Autodesk Inventor part; units mm, degrees
ref_plane "РабПлоскость1" through (0, 0, 75.2) normal (0, 0, 1) x (1, 0, 0)
ref_plane "YZ Plane" through (0, 0, 0) normal (1, 0, 0) x (0, 1, 0)
ref_plane "XZ Plane" through (0, 0, 0) normal (0, 1, 0) x (-1, 0, 0)
ref_plane "РабПлоскость1" through (0, 0, 75.2) normal (0, 0, 1) x (1, 0, 0)
sketch "Эскиз1" plane through (0, 0, 75.2) normal (0, 0, 1) x (1, 0, 0)
  circle A0 centre (26.4645, -26.4645) radius 1.95 construction
  circle A1 centre (-26.4645, 26.4645) radius 1.95 construction
  circle A2 centre (26.4645, 26.4645) radius 1.95 construction
  circle A3 centre (-26.4645, -26.4645) radius 1.95 construction
  circle A4 centre (15.35, -15.35) radius 1.7 construction
  circle A5 centre (-15.35, 15.35) radius 1.7 construction
  circle A6 centre (15.35, 15.35) radius 1.7 construction
  circle A7 centre (-15.35, -15.35) radius 1.7 construction
  line L0 (-32.5, 27.5) -> (-32.5, -27.5)
  line L1 (-27.5, 32.5) -> (-32.5, 27.5)
  line L2 (27.5, 32.5) -> (-27.5, 32.5)
  line L3 (32.5, 27.5) -> (27.5, 32.5)
  line L4 (32.5, -27.5) -> (32.5, 27.5)
  line L5 (27.5, -32.5) -> (32.5, -27.5)
  line L6 (-27.5, -32.5) -> (27.5, -32.5)
  line L7 (-32.5, -27.5) -> (-27.5, -32.5)
  circle A8 centre (0, 0) radius 11.5 construction
  circle A9 centre (0, 0) radius 26.7
  point P0 (0, 0)
extrude "Выдавливание1" add sketch "Эскиз1" along normal blind 4
sketch "Эскиз2" plane through (0, 0, 79.2) normal (0, 0, 1) x (1, 0, 0)
  circle A0 centre (26.4645, 26.4645) radius 2.25
  circle A1 centre (26.4645, -26.4645) radius 2.25
  circle A2 centre (-26.4645, -26.4645) radius 2.25
  circle A3 centre (-26.4645, 26.4645) radius 1.95
hole "Отверстие1" at (26.4645, 26.4645, 79.2) at (-26.4645, 26.4645, 79.2) at (26.4645, -26.4645, 79.2) at (-26.4645, -26.4645, 79.2) direction (0, 0, -1) diameter 3.4 end through all countersink diameter 6.6 countersink angle 90
properties part number "Крышка" material "По умолчанию1"
Verification items for the finished model (mm, model axes). Give positions to 0.01 mm unless a question says otherwise; leave off trailing zeros. Loops run counter-clockwise (first coordinate to the right, second up) from the corner with the lowest first, then second, coordinate; pieces in that order, holes last.
1. Go/stop test with a flat-tipped pin: pin 1 Ø12 at (x, y) = (-8.5, 17) entering from -Z. Record where the tip stops, or that it passes through.
2. Section check A-A, the plane x = 0. Enter the section's corners in (y, z).
3. Section check C-C, the plane z = 78.45. Enter the section's corners in (x, y), then the cut area to 3 significant figures.
4. Thickness scan on line 1 (Y direction, x = 0, z = 79); line 2 (Y direction, x = 28, z = 78.1); line 3 (Y direction, x = -28, z = 76.5). Record the ranges inside material, lowest first.
5. Mould release check, pull along X, two halves, no side actions. Record for faces 1 (the flat face through (32.5, 0, 77)), 2 (the cylindrical face through (25.467, -8.02, 77.172)), 3 (the flat face through (-30, 30, 77)): released by +X, released by -X, zero draft, split by the parting line, or undercut.
Geometry says:
1. pin 1: passes through
2. outline: (-32.5, 75.2) - (-26.7, 75.2) - (-26.7, 79.2) - (-32.5, 79.2) - close; (26.7, 75.2) - (32.5, 75.2) - (32.5, 79.2) - (26.7, 79.2) - close
3. outline: (-32.5, -27.5) - (-27.5, -32.5) - (27.5, -32.5) - (32.5, -27.5) - (32.5, 27.5) - (27.5, 32.5) - (-27.5, 32.5) - (-32.5, 27.5) - close; hole circle Ø5.1 at (-26.46, -26.46); hole circle Ø5.1 at (-26.46, 26.46); hole circle Ø53.4 at (0, 0); hole circle Ø5.1 at (26.46, -26.46); hole circle Ø5.1 at (26.46, 26.46)
3. area: 1,850 mm2
4. line 1: y = -32.5 to -26.7, 26.7 to 32.5
4. line 2: y = -32 to -28.04, -24.89 to 24.89, 28.04 to 32
4. line 3: y = -32 to -27.19, -25.73 to 25.73, 27.19 to 32
5. face 1: released by +X
5. face 2: undercut
5. face 3: released by -X
